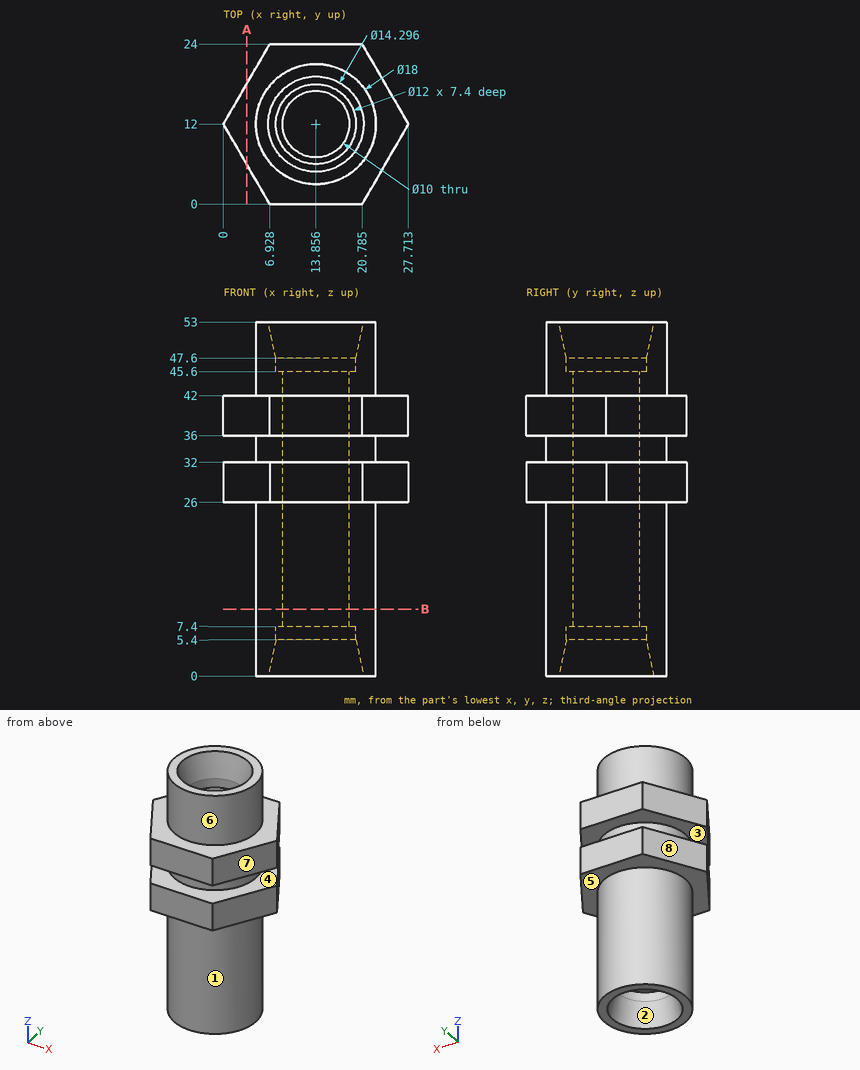
Part print with two shaded views. Sizes in mm from the minimum x, y, z corner. A direction names the side the tool comes from. Round coordinates to 2 decimals unless told otherwise and drop trailing zeros. Order: outer loops, then holes, each group sorted by start corner. A loop starts at its lowest first (then second) coordinate and runs counter-clockwise, first axis right, second up. Notation, with made-up numbers: (73.25, 22.5) - (98.25, 22.5) arc R19 ccw to (98.25, 51.5) - close; hole circle Ø6 at (40, 84.5). An arc over 180 degrees is marked (long way). Return JSON: item names as keys, results as strings.
(1) Wall check: probe 1 along Z at (x, y) = (25.75, 13.5); probe 2 along Z at (x, y) = (19, 12); probe 3 along Y at (x, z) = (24.25, 28) (1 decimal). Give the ranges that are in metal, low to high. Write a range as from..to.
Answer key:
{"probe 1": "z = 26..32, 36..42", "probe 2": "z = 7.4..45.6", "probe 3": "y = 6..18"}
(2) Tool access for the marked faces 4, 5, 6, 7 and 8: list every direction of +Z, -Z, +X, -X, +Y, -Y with a clear straight run to the whole face (end or side of a thin tool).
Answer key:
{"face 4": "none", "face 5": "-Z", "face 6": "+Z", "face 7": "+Z, -Z, +X, -Y", "face 8": "+Z, -Z, -X, +Y"}
(3) Cut at B-B (z = 10). Give the cut face in (x, y), then the cut area to 3 significant figures.
Answer key:
{"outline": "circle Ø18 at (13.86, 12); hole circle Ø10 at (13.86, 12)", "area": "176 mm^2"}
(4) Pull direction Y, two halves, no side cores. Call the marked faces 1, 2 and 3: +Y half, -Y half, draft (parallel to the pull), parting line (faces both ways), or undercut.
Answer key:
{"face 1": "parting line", "face 2": "undercut", "face 3": "draft"}
(5) Cut at A-A (x = 3.5). Give the cut face in (y, z).
Answer key:
{"outline": "(5.94, 26) - (18.06, 26) - (18.06, 32) - (5.94, 32) - close; (5.94, 36) - (18.06, 36) - (18.06, 42) - (5.94, 42) - close"}
(6) Pin check, flat tips, straight feed: pin 1 Ø8 at (y, z) = (21, 41) entering from -X; pin 2 Ø12 at (y, z) = (20.5, 25.5) entering from -X (1 decimal); pin 3 Ø1 at (y, z) = (10, 15.5) entering from -X; pin 4 Ø9.5 at (x, y) = (13.86, 12) entering from -Z. Stop position of each tip, or through.
Answer key:
{"pin 1": "stops at x = 2.89", "pin 2": "stops at x = 1.5", "pin 3": "stops at x = 4.98", "pin 4": "passes through"}
